```python
from build123d import *

# Parameters (mm, degrees)
SKETCH_R         = 1.4986
PAD_DEPTH        = 0.762
SKETCH001_R      = 1.3589
PAD001_DEPTH     = 0.7112
SKETCH002_R      = 1.2954
PAD002_DEPTH     = 4.5212
REVOLUTION_ANGLE = -180


with BuildPart() as part:
    # Sketch → Pad (new body)
    with BuildSketch(Plane.XY):
        Circle(SKETCH_R)
    extrude(amount=PAD_DEPTH)

    # Sketch001 (on Face3 of Pad) → Pad001 (join)
    with BuildSketch(Plane.XY.offset(0.762)):
        Circle(SKETCH001_R)
    extrude(amount=PAD001_DEPTH)

    # Sketch002 (on Face5 of Pad001) → Pad002 (join)
    with BuildSketch(Plane.XY.offset(1.4732)):
        Circle(SKETCH002_R)
    extrude(amount=PAD002_DEPTH)

    # Sketch003 (on Face7 of Pad002) → Revolution (revolve)
    with BuildSketch(Plane.XY.offset(5.9944)):
        with BuildLine():
            ThreePointArc((0, -1.1557), (1.1557, 0), (0, 1.1557))
            Line((0, 1.1557), (0, -1.1557))
        make_face()
    revolve(axis=Axis((0, 0, 5.9944), (0, 1, 0)), revolution_arc=REVOLUTION_ANGLE)


solid = part.part
```
The listing builds one solid part. Answer for the finished solid, in the listing's coordinates (mm). A direction names the side the tool comes from. Round coordinates to 2 decimals unless told otherwise and drop trailing zeros. Order: outer loops, then holes, each group sorted by start corner. A loop starts at its lowest first (then second) coordinate and runs counter-clockwise, first axis right, second up. Notation, with made-up numbers: (-37, 86.5) - (-17, 86.5) arc R11 cw to (-17, 96.5) - close; hole circle Ø6 at (23, -28). An arc over 180 degrees is marked (long way). Put each result on its own line as item: value. Start each with the question number.
(1) Find section A-A (x = 0). Give the vertices of the cut face in (y, z), plus the area to 3 significant figures.
(2) For faces 1 (the cylindrical face through (-0.281, -1.265, 3.702)), 2 (the cylindrical face through (1.43, 0.45, 0.38)), determine the directions among +Z, -Z, +X, -X, +Y, -Y from which every point of the face is accessible in a straight line to the end or side of a thin tool.
(3) Find section D-D (z = 6.5). Give the vertices of the cut face in (x, y), plus the area to 3 significant figures.
(4) Straight lines are drawn through the part: probe 1 along Z at (x, y) = (0, 1.45); probe 2 along X at (y, z) = (-0.05, 2); probe 3 along Z at (x, y) = (-1.15, 0.3). For each, find the intervals that lie inside material, in ascending order. Write a range as from..to.
(5) Find section C-C (z = 2.5). Give the vertices of the cut face in (x, y), plus the area to 3 significant figures.
(6) Given P1, Ø1, axis at y = 0.5, z = 3.5, coming from the +X side, flat-ended and moving along its own axis, determine where the tip first touches the part or whether it passes through.
Reply:
1. outline: (-1.5, 0) - (1.5, 0) - (1.5, 0.76) - (1.36, 0.76) - (1.36, 1.47) - (1.3, 1.47) - (1.3, 5.99) - (1.16, 5.99) arc R1.16 ccw to (-1.16, 5.99) - (-1.3, 5.99) - (-1.3, 1.47) - (-1.36, 1.47) - (-1.36, 0.76) - (-1.5, 0.76) - close
1. area: 18.0 mm^2
2. face 1: +Z
2. face 2: +Z, -Z
3. outline: circle Ø2.08 at (0, 0)
3. area: 3.39 mm^2
4. probe 1: 0..0.76
4. probe 2: -1.29..1.29
4. probe 3: 0..5.99
5. outline: circle Ø2.59 at (0, 0)
5. area: 5.27 mm^2
6. P1: x = 1.3
